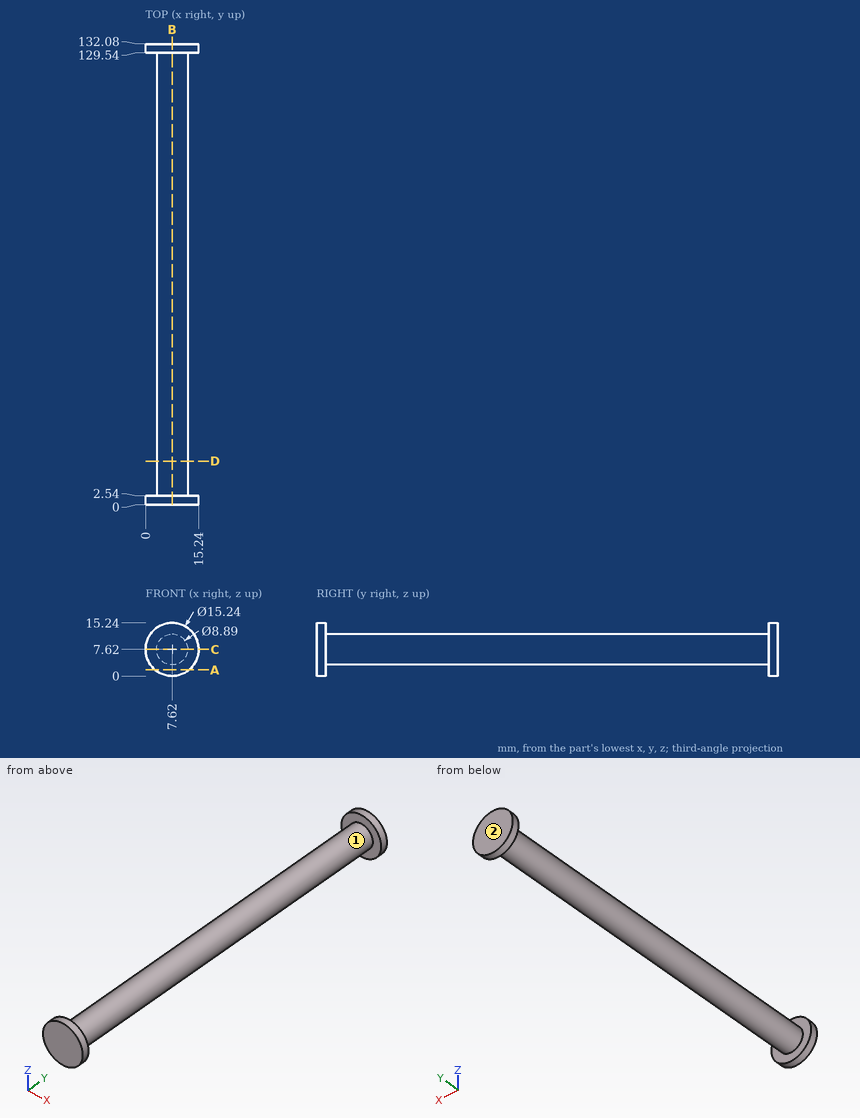
Geometry: see drawing. Coordinates: mm, zero at the bounding-box minimum. A direction names the side the tool comes from. Coordinates: 2 decimals unless noted, no trailing zeros. Write each loop counter-clockwise with the first axis right and the second up, starting at its lowest first coordinate (ties: lowest second). Pieces come first, ordered by that corner, then holes. Notation, with made-up numbers: M 29.5,29 L 68.5,29 A18 cw 68.5,37 Z; hole C 52,-36.75 d11. An arc over 180 degrees is marked long. Use CSV: the item, a comma, the result in double quotes. Start each with the question number.
1. Cut plane D-D on y = 12.5. Return the cut outline in (x, z) (3 decimals).
2. Cut plane C-C on z = 7.62. Return the cut outline in (x, y) (3 decimals), plus the area to 3 significant figures.
3. First-contact query: P1, Ø4, axis at x = 2, y = 89, coming from the -Z side; P2, Ø5, axis at y = 104.5, z = 7, coming from the -X side (3 decimals); P3, Ø1, axis at y = 40, z = 11, coming from the -X side. Flat tips, straight axial feed; report the tip coordinate or a pass-through.
4. Reachability of the marked faces 1 and 2 from +Z, -Z, +X, -X, +Y, -Y: full face, straight path, thin tool, end or side. Return the list, or none.
5. Cut plane A-A on z = 1.75. Return the cut outline in (x, y), plus the area to 3 significant figures.
6. Cut plane B-B on x = 7.62. Return the cut outline in (y, z) (3 decimals), plus the area to 3 significant figures.
7. Ray query, probe 1 along Y at (x, z) = (2.25, 6); probe 2 along X at (y, z) = (102.5, 8); probe 3 along X at (y, z) = (103.5, 11). Return the intervals inside material, ascending.
Entries:
1,outline,"C 7.62,7.62 d8.89"
2,outline,"M 0,0 L 15.24,0 L 15.24,2.54 L 12.065,2.54 L 12.065,129.54 L 15.24,129.54 L 15.24,132.08 L 0,132.08 L 0,129.54 L 3.175,129.54 L 3.175,2.54 L 0,2.54 Z"
2,area,"1,210 mm²"
3,P1,"z = 5.04"
3,P2,"x = 3.175"
3,P3,"x = 4.23"
4,face 1,"none"
4,face 2,"+Z, -Z, +X, -X, +Y"
5,outline,"M 2.76,0 L 12.48,0 L 12.48,2.54 L 2.76,2.54 Z; M 2.76,129.54 L 12.48,129.54 L 12.48,132.08 L 2.76,132.08 Z"
5,area,"49.4 mm²"
6,outline,"M 0,0 L 2.54,0 L 2.54,3.175 L 129.54,3.175 L 129.54,0 L 132.08,0 L 132.08,15.24 L 129.54,15.24 L 129.54,12.065 L 2.54,12.065 L 2.54,15.24 L 0,15.24 Z"
6,area,"1,210 mm²"
7,probe 1,"0 to 2.54, 129.54 to 132.08"
7,probe 2,"3.19 to 12.05"
7,probe 3,"4.73 to 10.51"
